Can you work these out from the model? Positions are in its coordinate system, mm. Give positions to 0.01 mm unless a question says otherwise; leave off trailing zeros. Order: outer loops, then holes, each group sorted by start corner. A loop starts at its lowest first (then second) coordinate and runs counter-clockwise, first axis right, second up. Notation, with made-up numbers: (88.5, 23.5) - (100.5, 23.5) arc R21 cw to (100.5, 30.5) - close; hole circle Ø5 at (21.25, 67). An arc over 180 degrees is marked (long way). Answer as CSV lines item,"result".
```python
from build123d import *

# Parameters (mm, degrees)
EXTRUDE_1_DEPTH = 1000


with BuildPart() as part:
    # Эскиз1 → Бобышка-Вытянуть1 (new body)
    with BuildSketch(Plane.XY):
        with BuildLine():
            Line((-3.1, 0), (-4, -0.158694283))
            Line((-4, -0.158694283), (-4, -0.8))
            Line((-4, -0.8), (-3.1, -0.8))
            Line((-3.1, -0.8), (-3.1, -2.196152423))
            Line((-3.1, -2.196152423), (-3.68771324, -3.214101615))
            Line((-3.68771324, -3.214101615), (-3.1, -4.232050808))
            ThreePointArc((-3.1, -4.232050808), (-2.497197677, -4.481739705), (-2.1, -3.964101615))
            Line((-2.1, -3.964101615), (-2.533012702, -3.214101615))
            Line((-2.533012702, -3.214101615), (-2.1, -2.464101615))
            Line((-2.1, -2.464101615), (-2.1, -1))
            Line((-2.1, -1), (2.1, -1))
            Line((2.1, -1), (2.1, -2.464101615))
            Line((2.1, -2.464101615), (2.533012702, -3.214101615))
            Line((2.533012702, -3.214101615), (2.1, -3.964101615))
            ThreePointArc((2.1, -3.964101615), (2.497197677, -4.481739705), (3.1, -4.232050808))
            Line((3.1, -4.232050808), (3.68771324, -3.214101615))
            Line((3.68771324, -3.214101615), (3.1, -2.196152423))
            Line((3.1, -2.196152423), (3.1, -0.8))
            Line((3.1, -0.8), (4, -0.8))
            Line((4, -0.8), (4, -0.158694283))
            Line((4, -0.158694283), (3.1, 0))
            Line((3.1, 0), (-3.1, 0))
        make_face()
    extrude(amount=EXTRUDE_1_DEPTH)


solid = part.part
```
1) I need wall thicknesses on line 1 along X through (y, z) = (-1.8, 137); line 2 along X through (y, z) = (-4.2, 954.5); line 3 along Y through (x, z) = (2.25, 914.5). Which ranges of each line are inside material? Lowest first, please. Write a range as [from, to].
Answer block:
line 1,"[-3.1, -2.1], [2.1, 3.1]"
line 2,"[-3.12, -2.15], [2.15, 3.12]"
line 3,"[-4.34, -3.7], [-2.72, 0]"
2) I want a section at A-A on z = 149. Write out the boundary of the cut face in (x, y).
Answer block:
outline,"(-4, -0.8) - (-3.1, -0.8) - (-3.1, -2.2) - (-3.69, -3.21) - (-3.1, -4.23) arc R0.54 ccw to (-2.1, -3.96) - (-2.53, -3.21) - (-2.1, -2.46) - (-2.1, -1) - (2.1, -1) - (2.1, -2.46) - (2.53, -3.21) - (2.1, -3.96) arc R0.54 ccw to (3.1, -4.23) - (3.69, -3.21) - (3.1, -2.2) - (3.1, -0.8) - (4, -0.8) - (4, -0.16) - (3.1, 0) - (-3.1, 0) - (-4, -0.16) - close"
3) I'm going to push flat-ended pins straight in: P1, Ø2, axis at x = 0.5, z = 599, coming from the -Y side; P2, Ø1.1, axis at y = -1.5, z = 724, coming from the +X side; P3, Ø1.2, axis at y = -2, z = 562, coming from the +X side; P4, Ø4, axis at x = 2.5, z = 485, coming from the +Y side. Where does each tip first touch, or does it pass through?
Answer block:
P1,"y = -1"
P2,"x = 3.1"
P3,"x = 3.33"
P4,"y = 0"
